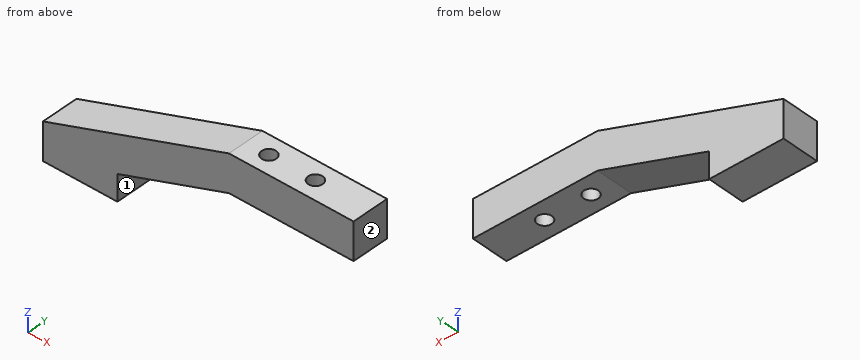
from build123d import *

# Parameters (mm, degrees)
SKETCH3_W           = 13.4
SKETCH3_H           = 4
SKETCH3_R           = 0.78
BOSS_EXTRUDE1_DEPTH = 4
BOSS_EXTRUDE2_DEPTH = 4
SKETCH5_W           = 8
SKETCH5_H           = 4
BOSS_EXTRUDE3_DEPTH = 1


with BuildPart() as part:
    # Sketch3 → Boss-Extrude1 (new body)
    with BuildSketch(Plane.XY):
        with Locations((6.7, 2)):
            Rectangle(SKETCH3_W, SKETCH3_H)
        with Locations((2.5, 2)):
            Circle(SKETCH3_R, mode=Mode.SUBTRACT)
        with Locations((7.5, 2)):
            Circle(SKETCH3_R, mode=Mode.SUBTRACT)
    extrude(amount=BOSS_EXTRUDE1_DEPTH)

    # Sketch4 → Boss-Extrude2 (add)
    with BuildSketch(Plane(origin=(0, 4, 0), x_dir=(1, 0, 0), z_dir=(0, 1, 0))):
        Polygon((0, -4), (-20, 3), (-20, 6), (-12, 6), (-12, 4.2), (0, 0), align=None)
    extrude(amount=-BOSS_EXTRUDE2_DEPTH)

    # Sketch5 → Boss-Extrude3 (add)
    with BuildSketch(Plane(origin=(0, 0, -6), x_dir=(-1, 0, 0), z_dir=(0, 0, -1))):
        with Locations((16, 2)):
            Rectangle(SKETCH5_W, SKETCH5_H)
    extrude(amount=BOSS_EXTRUDE3_DEPTH)


solid = part.part
Could you check a few things on this model? Use its own coordinates, in mm. Face numbers are marked on the shaded views. A direction names the side the tool comes from. Give positions to 0.01 mm unless a question says otherwise; leave off trailing zeros. Order: outer loops, then holes, each group sorted by start corner. A loop starts at its lowest first (then second) coordinate and runs counter-clockwise, first axis right, second up. Notation, with made-up numbers: (-11, 87.25) -> (-2, 87.25) arc R27 ccw to (-2, 123.25) -> close; hole circle Ø3 at (71, 89.5). An arc over 180 degrees is marked (long way). Return JSON: item names as keys, results as strings.
1. Imagine slicing it at D-D on y = 0.4. List the corners of the cut face in (x, z) for me, then the cut area to 3 significant figures.
Answer list:
{"outline": "(-20, -7) -> (-12, -7) -> (-12, -4.2) -> (0, 0) -> (13.4, 0) -> (13.4, 4) -> (0, 4) -> (-20, -3) -> close", "area": "145 mm2"}
2. Imagine slicing it at A-A on x = 7.5. List the corners of the cut face in (y, z) for me, then the cut area to 3 significant figures.
Answer list:
{"outline": "(0, 0) -> (1.22, 0) -> (1.22, 4) -> (0, 4) -> close; (2.78, 0) -> (4, 0) -> (4, 4) -> (2.78, 4) -> close", "area": "9.76 mm2"}
3. For pin 1 Ø1.5 at (x, y) = (9, 2.5) entering from -Z; pin 2 Ø1 at (x, y) = (-1.5, 0.5) entering from +Z; pin 3 Ø1.5 at (x, y) = (-4.5, 1) entering from -Z, each with a flat end and sliding along its axis, tell me the tip position at first contact or that it passes through.
Answer list:
{"pin 1": "stops at z = 0", "pin 2": "stops at z = 3.65", "pin 3": "stops at z = -1.84"}
4. On a 3-axis mill with a long thin cutter (end or side, diameter ignored), from which of +Z, -Z, +X, -X, +Y, -Y can I reach the whole of each face in a straight line? I mean the marked faces 1 and 2. Say none if no direction works.
Answer list:
{"face 1": "-Z, +X, +Y, -Y", "face 2": "+Z, -Z, +X, +Y, -Y"}
5. Imagine slicing it at C-C on z = 0.5. List the corners of the cut face in (x, y) for me.
Answer list:
{"outline": "(-10, 0) -> (13.4, 0) -> (13.4, 4) -> (-10, 4) -> close; hole circle Ø1.56 at (2.5, 2); hole circle Ø1.56 at (7.5, 2)"}
6. Imagine slicing it at B-B on y = 2. List the corners of the cut face in (x, z) for me.
Answer list:
{"outline": "(-20, -7) -> (-12, -7) -> (-12, -4.2) -> (0, 0) -> (1.72, 0) -> (1.72, 4) -> (0, 4) -> (-20, -3) -> close; (3.28, 0) -> (6.72, 0) -> (6.72, 4) -> (3.28, 4) -> close; (8.28, 0) -> (13.4, 0) -> (13.4, 4) -> (8.28, 4) -> close"}
7. I need wall thicknesses on line 1 (Y direction, x = 7.5, z = 0.95); line 2 (Z direction, x = 1, y = 1.6); line 3 (X direction, y = 0.4, z = -4.25). Which ranges of each line are inside material? Lowest first, please. Write a range as from..to.
Answer list:
{"line 1": "y = 0..1.22, 2.78..4", "line 2": "z = 0..4", "line 3": "x = -20..-12"}
